from build123d import *

# Parameters (mm, degrees)
F0_R         = 2.54
F1_DEPTH     = 18.25625
F2_W         = 7.9375
F2_H         = 7.9375
F3_DEPTH     = 7.9375
F4_R         = 3.96875
F5_DEPTH     = 7.9375
F6_T1_DEPTH  = 27.78125
F6_T6_DEPTH  = 27.78125
F6_S7_R      = 2.54
F6_T8_DEPTH  = 16
F6_T12_DEPTH = 27.78125
F6_S13_R     = 2.54
F6_T14_DEPTH = 16
F7_R         = 2.54
F8_DEPTH     = 7.9375


# Not quite as in the source:
# - a fillet or chamfer that OpenCascade refuses, or shapes differently, is made with other operations: its cross-section is extruded or revolved along the edge and cut away or added


with BuildPart() as f1:
    # F0 (on Top) → F1 (new body)
    with BuildSketch(Plane.XY):
        Circle(F0_R)
    extrude(amount=F1_DEPTH)

    # F2 (on face) → F3 (join)
    with BuildSketch(Plane(origin=(0, 0, 0), x_dir=(1, 0, 0), z_dir=(0, 0, -1))):
        Rectangle(F2_W, F2_H)
    extrude(amount=F3_DEPTH)

    # F4 (on face) → F5 (join)
    with BuildSketch(Plane.XY.offset(18.25625)):
        Circle(F4_R)
    extrude(amount=F5_DEPTH)

    # F6: fillet of radius 3.96875 on 4 edges, made by hand

    # F6_s2 → F6_t1 (cut)
    with BuildSketch(Plane.YZ.offset(-13.890625)):
        with BuildLine():
            ThreePointArc((3.96875, -3.96875), (2.8063300378, -6.7750800378), (0, -7.9375))
            Line((0, -7.9375), (3.96875, -7.9375))
            Line((3.96875, -7.9375), (3.96875, -3.96875))
        make_face()
        with BuildLine():
            ThreePointArc((-3.96875, -3.96875), (-2.8063300378, -6.7750800378), (0, -7.9375))
            Line((0, -7.9375), (-3.96875, -7.9375))
            Line((-3.96875, -7.9375), (-3.96875, -3.96875))
        make_face()
    extrude(amount=F6_T1_DEPTH, mode=Mode.SUBTRACT)


with BuildPart() as f6_tool4:
    # F6_s5 → F6_t6 (new body)
    with BuildSketch(Plane.YZ.offset(13.890625)):
        with BuildLine():
            ThreePointArc((0, 0), (-2.8063300378, -1.1624199622), (-3.96875, -3.96875))
            Line((-3.96875, -3.96875), (-3.96875, 0))
            Line((-3.96875, 0), (0, 0))
        make_face()
    extrude(amount=-F6_T6_DEPTH)

    # F6_s7 → F6_t8 (cut, symmetric)
    with BuildSketch(Plane.XY.offset(-2)):
        Circle(F6_S7_R)
    extrude(amount=F6_T8_DEPTH, both=True, mode=Mode.SUBTRACT)


with BuildPart() as f1_1:
    add(f1.part)

    # F6_t3: cut F6_tool4
    add(f6_tool4.part, mode=Mode.SUBTRACT)


with BuildPart() as f6_tool10:
    # F6_s11 → F6_t12 (new body)
    with BuildSketch(Plane.YZ.offset(-13.890625)):
        with BuildLine():
            ThreePointArc((0, 0), (2.8063300378, -1.1624199622), (3.96875, -3.96875))
            Line((3.96875, -3.96875), (3.96875, 0))
            Line((3.96875, 0), (0, 0))
        make_face()
    extrude(amount=F6_T12_DEPTH)

    # F6_s13 → F6_t14 (cut, symmetric)
    with BuildSketch(Plane.XY.offset(-2)):
        Circle(F6_S13_R)
    extrude(amount=F6_T14_DEPTH, both=True, mode=Mode.SUBTRACT)


with BuildPart() as f1_2:
    add(f1_1.part)

    # F6_t9: cut F6_tool10
    add(f6_tool10.part, mode=Mode.SUBTRACT)

    # F7 (on face) → F8 (cut, through all)
    with BuildSketch(Plane(origin=(-3.96875, 0, 0), x_dir=(0, -1, 0), z_dir=(-1, 0, 0))):
        with Locations((0, -3.96875)):
            Circle(F7_R)
    extrude(amount=-F8_DEPTH, mode=Mode.SUBTRACT)


solid = f1_2.part
Geometry check sheet. Reference: the model listing, model coordinates, mm. A direction names the side the tool comes from. Give positions to 0.01 mm unless a question says otherwise; leave off trailing zeros. Write each loop counter-clockwise with the first axis right and the second up, starting at its lowest first coordinate (ties: lowest second). Pieces come first, ordered by that corner, then holes.
1) Cross-section at C-C (y = -1). Record the boundary of the cut face in (x, z), plus the area to 3 significant figures.
Values follow:
outline: (-3.97, -7.81) - (3.97, -7.81) - (3.97, -6.3) - (-3.97, -6.3) - close; (-3.97, -1.63) - (3.97, -1.63) - (3.97, -0.13) - (2.33, -0.13) - (2.33, 18.26) - (3.84, 18.26) - (3.84, 26.19) - (-3.84, 26.19) - (-3.84, 18.26) - (-2.33, 18.26) - (-2.33, -0.13) - (-3.97, -0.13) - close
area: 171 mm2
2) Release check for a two-part mould opening along Z. For faces 3 (the face through (-3.969, 0, -7)), 4 (the face through (0, 0, 26.194)), 5 (the face through (0, -3, 18.256)), 6 (the face through (-0.33, 2.52, 8.53)) record: released by +Z, released by -Z, zero draft, split by the parting line, or undercut.
Values follow:
face 3: zero draft
face 4: released by +Z
face 5: undercut
face 6: undercut
3) Set-up check for faces 1 (the face through (-0.86, -3.874, 22.169)), 2 (the face through (-0.06, 0.33, -1.45)): record each of +Z, -Z, +X, -X, +Y, -Y from which the full face is reachable in a straight line by a thin tool's end or side.
Values follow:
face 1: +Z
face 2: +X, -X
4) Cross-section at A-A (x = 3.25). Record the boundary of the cut face in (y, z), plus the area to 3 significant figures.
Values follow:
outline: circle Ø7.94 at (0, -3.97); (-2.28, 18.26) - (2.28, 18.26) - (2.28, 26.19) - (-2.28, 26.19) - close; hole circle Ø5.08 at (0, -3.97)
area: 65.4 mm2
5) Thickness scan on line 1 (Z direction, x = 0.25, y = 0); line 2 (Z direction, x = -2.5, y = -1); line 3 (Z direction, x = 2.5, y = 2). Record the ranges inside material, lowest first.
Values follow:
line 1: z = -7.94 to -6.51, -1.43 to 26.19
line 2: z = -7.81 to -6.3, -1.63 to -0.13, 18.26 to 26.19
line 3: z = -7.4 to -5.53, -2.4 to -0.54, 18.26 to 26.19
6) Cross-section at B-B (x = 0). Record the boundary of the cut face in (y, z).
Values follow:
outline: (-3.97, 18.26) - (-2.54, 18.26) - (-2.54, -0.92) arc R3.97 ccw (long way) to (2.54, -0.92) - (2.54, 18.26) - (3.97, 18.26) - (3.97, 26.19) - (-3.97, 26.19) - close; hole circle Ø5.08 at (0, -3.97)
7) Go/stop test with flat-tipped pins: pin 1 Ø1.5 at (x, z) = (1, -1) entering from +Y; pin 2 Ø1.5 at (y, z) = (1, 9.5) entering from -X. Record where each tip stops, or that it passes through.
Values follow:
pin 1: stops at y = 3.29
pin 2: stops at x = -2.53
8) Cross-section at D-D (z = -2). Record the boundary of the cut face in (x, y).
Values follow:
outline: (-3.97, -3.45) - (3.97, -3.45) - (3.97, -1.6) - (-3.97, -1.6) - close; (-3.97, 1.6) - (3.97, 1.6) - (3.97, 3.45) - (-3.97, 3.45) - close
